Autodesk Inventor part; units mm, degrees
ref_plane "Work Plane1" through (0, 160, 0) normal (0, 1, 0) x (-1, 0, 0)
ref_plane "Work Plane2" through (0, 80, 0) normal (0, 1, 0) x (-1, 0, 0)
ref_plane "YZ Plane" through (0, 0, 0) normal (1, 0, 0) x (0, 1, 0)
sketch "Sketch1" plane through (0, 0, 0) normal (0, 1, 0) x (-1, 0, 0)
  circle A0 centre (0, 0) radius 63.5
  circle A1 centre (0, 0) radius 66.5
  dimension "d0" = 127
  dimension "d1" = 133
extrude "Extrusion1" add sketch "Sketch1" along normal blind 160
ref_plane "Work Plane1" through (0, 160, 0) normal (0, 1, 0) x (-1, 0, 0)
sketch "Sketch2" plane through (0, 160, 0) normal (0, 1, 0) x (-1, 0, 0)
  circle A0 centre (0, 0) radius 63.5
  dimension "d5" = 127
extrude "Extrusion2" add sketch "Sketch2" against normal blind 3
chamfer "Chamfer1" distance 5 angle 45 1 edges at (66.5, 160, 0)
chamfer "Chamfer2" distance 5 angle 45 1 edges at (63.5, 157, 0)
ref_plane "Work Plane2" through (0, 80, 0) normal (0, 1, 0) x (-1, 0, 0)
sketch "Sketch3" plane through (0, 80, 0) normal (0, 1, 0) x (-1, 0, 0)
  circle A0 centre (0, 0) radius 63.5
  circle A1 centre (0, 0) radius 66.5
  line L0 (0, 0) -> (0, -66.5)
  line L1 (0, 0) -> (33.25, -57.5907)
  line L2 (0, 0) -> (66.5, 0) construction
  line L3 (0, 0) -> (0, 66.5)
  line L4 (0, 0) -> (-33.25, 57.5907)
  point P0 (0, 63.5)
  point P1 (31.75, -54.9926)
  point P2 (-31.75, 54.9926)
  point P3 (0, -63.5)
  dimension "d15" = 127
  dimension "d16" = 133
  dimension "d17" = 60
extrude "Extrusion3" cut sketch "Sketch3" along normal blind 40 contours A0 L3 A1 L1 | A0 L0 A1 L4
properties part number "siren_new" material "ABS Plastic"
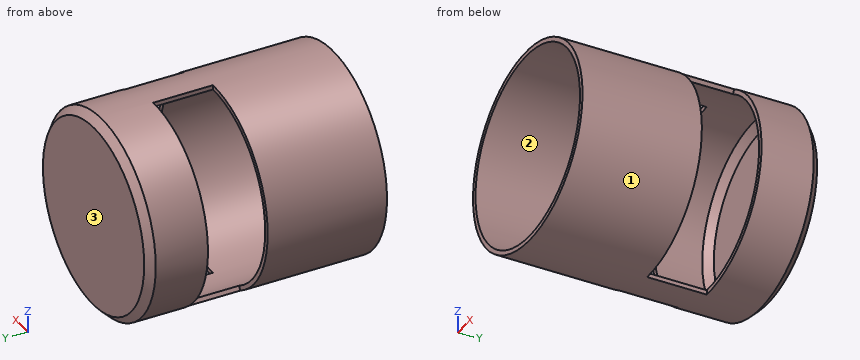
Can you work these out from the model? Positions are in its coordinate system, mm. Face numbers are marked on the shaded views. Give positions to 0.01 mm unless a question says otherwise; leave off trailing zeros. Order: outer loops, then holes, each group sorted by start corner. A loop starts at its lowest first (then second) coordinate and runs counter-clockwise, first axis right, second up. Notation, with made-up numbers: M 48.5,18 L 76.5,18 A18 cw 76.5,32 Z; hole C -11,75.25 d2. An arc over 180 degrees is marked long. Use a Markdown table: item, result. Add a question column.
Item 1: If I drill on L1, parallel to Z at x = 0, y = 72; L2, parallel to Z at x = -1.5, y = 87, over which ranges is the centre line in solid material (lowest first)? Write a range as [from, to].
Item 2: Suppose I cut it at D-D (y = 18). List the corners of the cut face in (x, z) for me.
Item 3: We'd pull the mould along X, two halves only. Please class the marked faces 1, 2 and 3: +X half, -X half, draft (parallel to the pull), parting line (faces both ways), or undercut.
Item 4: Suppose I cut it at C-C (x = -41). Count the separate pieces of the cut face and the enclosed holes in it, then the cut area to 3 significant figures.
Item 5: Suppose I cut it at A-A (y = 82). List the corners of the cut face in (x, z) for me, then the cut area to 3 significant figures.
Item 6: Suppose I cut it at B-B (z = 0). List the corners of the cut face in (x, y) for me.
Item 7: Will these pins go through, and if not, where does the flat tip stop? pin 1 (4 mm diameter, centred on x = -12.5, z = -25, fed in from -Y); pin 2 (12 mm diameter, centred on y = 82, z = 11.5, fed in from +X); pin 3 (5 mm diameter, centred on x = -19.5, y = 64, fed in from +Z).
Answer sheet:
| question | item | result |
|---|---|---|
| 1 | L1 | z = [-66.5, -63.5], [63.5, 66.5] |
| 1 | L2 | z = [-66.48, -63.48] |
| 2 | outline | C 0,0 d133; hole C 0,0 d127 |
| 3 | face 1 | parting line |
| 3 | face 2 | undercut |
| 3 | face 3 | draft |
| 4 | separate pieces | 3 |
| 4 | enclosed holes | 0 |
| 4 | area | 1,220 mm² |
| 5 | outline | M -33.25,-57.59 A66.5 ccw 0,-66.5 L 0,-63.5 A63.5 cw -31.75,-54.99 Z; M 0,63.5 A63.5 cw 31.75,54.99 L 33.25,57.59 A66.5 ccw 0,66.5 Z |
| 5 | area | 204 mm² |
| 6 | outline | M -66.5,0 L -63.5,0 L -63.5,80 L -66.5,80 Z; M -66.5,120 L -63.5,120 L -63.5,152 L -58.5,157 L 58.5,157 L 63.5,152 L 63.5,120 L 66.5,120 L 66.5,155 L 61.5,160 L -61.5,160 L -66.5,155 Z; M 63.5,0 L 66.5,0 L 66.5,80 L 63.5,80 Z |
| 7 | pin 1 | stops at y = 157 |
| 7 | pin 2 | stops at x = 66.24 |
| 7 | pin 3 | stops at z = 64.29 |
